Autodesk Inventor part; units mm, degrees
ref_plane "YZ Plane" through (0, 0, 0) normal (1, 0, 0) x (0, 1, 0)
ref_plane "XZ Plane" through (0, 0, 0) normal (0, 1, 0) x (-1, 0, 0)
ref_plane "XY Plane" through (0, 0, 0) normal (0, 0, 1) x (1, 0, 0)
sketch "スケッチ1" plane through (0, 0, 0) normal (0, 0, 1) x (1, 0, 0)
  circle A0 centre (0, 0) radius 2
  dimension "d0" = 4
extrude "押し出し1" add sketch "スケッチ1" along normal blind 6
sketch "スケッチ2" plane through (0, 0, 6) normal (0, 0, 1) x (1, 0, 0)
  circle A0 centre (0, 0) radius 2
  circle A1 centre (0, 0) radius 4
  dimension "d3" = 8
extrude "押し出し2" add sketch "スケッチ2" along normal blind 3 contours A0 | A1
fillet "フィレット1" radius 3 1 edges at (-4, 0, 9)
thread "ねじ1"
sketch "スケッチ3" plane through (0, 0, 0) normal (0, 0, -1) x (-1, 0, 0)
  circle A0 centre (0, 0) radius 2
extrude "押し出し3" add sketch "スケッチ3" along normal blind 4
properties part number "SB　M4 10mm なべネジ" material "Stainless Steel, 440C"
Can you work these out from the model? Positions are in its coordinate system, mm. A direction names the side the tool comes from. Round coordinates to 2 decimals unless told otherwise and drop trailing zeros. Loops run counter-clockwise (first coordinate to the right, second up) from the corner with the lowest first, then second, coordinate; pieces in that order, holes last. Notation, with made-up numbers: M 4,71 L 26,71 A21 cw 26,76 Z; hole C -16,61.5 d10. An arc over 180 degrees is marked long. Write item = value, one per line. Start each with the question number.
(1) I'm going to push flat-ended pins straight in: P1, Ø1.5, axis at y = -0.5, z = 4, coming from the +X side; P2, Ø4, axis at x = -2.5, y = 0, coming from the +Z side. Where does each tip first touch, or does it pass through?
(2) Suppose I cut it at A-A on z = 4. Write out the boundary of the cut face in (x, y).
(3) I need wall thicknesses on line 1 along X through (y, z) = (0, -1.25); line 2 along Y through (x, z) = (-0.25, 6.5); line 3 along Z through (x, y) = (1.75, 1.25). Which ranges of each line are inside material? Lowest first, please.
(4) Which directions (+Z, -Z, +X, -X, +Y, -Y) give clear straight access to the entire face, cutting with the end or side of a thin tool? Please do faces 1 (the face through (0, 0, 9)), 2 (the face through (-2, -1, 6)).
Answer block:
q1.P1 = 2
q1.P2 = 9
q2.outline = C 0,0 d4
q3.line_1 = -2 to 2
q3.line_2 = -3.95 to 3.95
q3.line_3 = 6 to 8.77
q4.face_1 = +Z, +X, -X, +Y, -Y
q4.face_2 = -Z
